Job drawing, mm, ordinate dimensions from the low corner. One solid piece. A direction names the side the tool comes from. Round coordinates to 2 decimals unless told otherwise and drop trailing zeros. Write each loop counter-clockwise with the first axis right and the second up, starting at its lowest first coordinate (ties: lowest second). Pieces come first, ordered by that corner, then holes.
1) Flat gauge pins, fed straight in: pin 1 (12.5 mm diameter, centred on x = 24, y = 26.5, fed in from -Z); pin 2 (1 mm diameter, centred on y = 31.5, z = 3, fed in from -X); pin 3 (4 mm diameter, centred on y = 16, z = 6, fed in from +X). Where does each tip first touch, or does it go through?
2) Wall check: probe 1 along Y at (x, z) = (13.5, 1.5); probe 2 along Z at (x, y) = (22.5, 24.5); probe 3 along Y at (x, z) = (10, 5.25). Give the ranges that are in metal, low to high.
3) Saw through at D-D (y = 13). Write the cut outline in (x, z), plus the area to 3 significant figures.
4) Which spindle directions (+Z, -Z, +X, -X, +Y, -Y) get a long thin tool onto all of the face, cutting with end or side? Do the marked faces 4, 5 and 6. Say none if no direction does.
5) Saw through at A-A (x = 12). Write the cut outline in (y, z), plus the area to 3 significant figures.
6) Pull direction Y, two halves, no side cores. Call the marked faces 1, 2 and 3: +Y half, -Y half, draft (parallel to the pull), parting line (faces both ways), or undercut.
7) Saw through at B-B (z = 6.25). Write the cut outline in (x, y).
8) Saw through at C-C (x = 17). Write the cut outline in (y, z), plus the area to 3 significant figures.
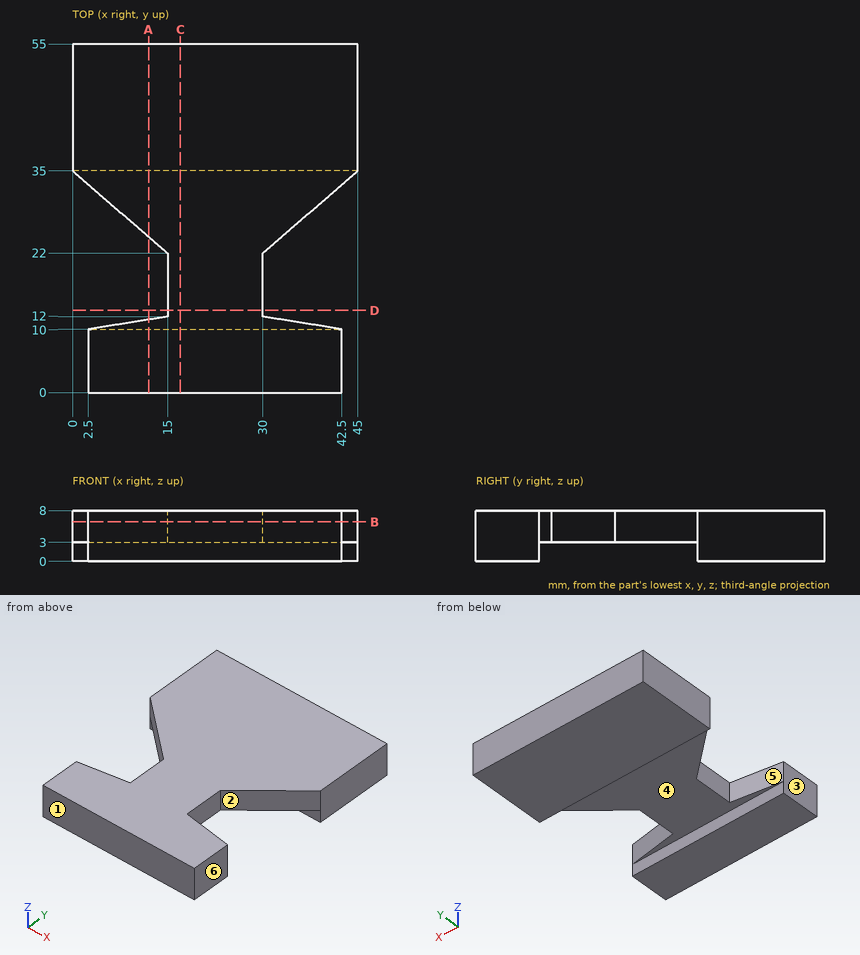
Evaluation:
1. pin 1: stops at z = 3
1. pin 2: stops at x = 3.46
1. pin 3: stops at x = 30
2. probe 1: y = 0 to 10, 35 to 55
2. probe 2: z = 3 to 8
2. probe 3: y = 0 to 11.2, 26.33 to 55
3. outline: (15, 3) - (30, 3) - (30, 8) - (15, 8) - close
3. area: 75.0 mm2
4. face 4: -Z, +X, -X
4. face 5: +Z, -Z, -X
4. face 6: +Z, -Z, +X, -Y
5. outline: (0, 0) - (10, 0) - (10, 3) - (11.52, 3) - (11.52, 8) - (0, 8) - close; (24.6, 3) - (35, 3) - (35, 0) - (55, 0) - (55, 8) - (24.6, 8) - close
5. area: 300 mm2
6. face 1: -Y half
6. face 2: undercut
6. face 3: draft
7. outline: (0, 35) - (15, 22) - (15, 12) - (2.5, 10) - (2.5, 0) - (42.5, 0) - (42.5, 10) - (30, 12) - (30, 22) - (45, 35) - (45, 55) - (0, 55) - close
8. outline: (0, 0) - (10, 0) - (10, 3) - (35, 3) - (35, 0) - (55, 0) - (55, 8) - (0, 8) - close
8. area: 365 mm2
